Geometry check sheet. Reference: the model listing, model coordinates, mm. A direction names the side the tool comes from. Give positions to 0.01 mm unless a question says otherwise; leave off trailing zeros. Write each loop counter-clockwise with the first axis right and the second up, starting at its lowest first coordinate (ties: lowest second). Pieces come first, ordered by that corner, then holes. Notation, with made-up numbers: (81, 65.5) - (129, 65.5) arc R23 cw to (129, 88.5) - close; hole circle Ø2 at (71, 57.5). An arc over 180 degrees is marked (long way). Use a Markdown table: item, result.
```python
from build123d import *

# Parameters (mm, degrees)
CROQUIS1_R              = 4
CROQUIS1_R_2            = 2.5
CROQUIS1_R_3            = 1.5
SALIENTE_EXTRUIR1_DEPTH = 5.5
CORTAR_EXTRUIR1_DEPTH   = 10
REDONDEO1_R             = 10


with BuildPart() as part:
    # Croquis1 → Saliente-Extruir1 (new body)
    with BuildSketch(Plane.XY):
        with BuildLine():
            ThreePointArc((13.175908043, 16.287969402), (20.207859701, 17.03070481), (19.465124293, 24.062656467))
            Line((19.465124293, 24.062656467), (1.886764875, 38.28240612))
            ThreePointArc((1.886764875, 38.28240612), (1.000695169, 38.778181249), (0, 38.95))
            Line((0, 38.95), (-14, 38.95))
            ThreePointArc((-14, 38.95), (-15.75421382, 38.383666755), (-16.84611457, 36.898489248))
            Line((-16.84611457, 36.898489248), (-19.121320344, 30.071320344))
            ThreePointArc((-19.121320344, 30.071320344), (-19.771638598, 29.098050297), (-20, 27.95))
            Line((-20, 27.95), (-20, 23.95))
            ThreePointArc((-20, 23.95), (-19.121320344, 21.828679656), (-17, 20.95))
            Line((-17, 20.95), (-5, 20.95))
            ThreePointArc((-5, 20.95), (-0.298863721, 15.958939945), (4.964272191, 20.353341289))
            ThreePointArc((4.964272191, 20.353341289), (9.295071106, 18.775093958), (13.175908043, 16.287969402))
        make_face()
        with Locations((0, 20.95)):
            Circle(CROQUIS1_R, mode=Mode.SUBTRACT)
        with Locations((-15, 25.95)):
            Circle(CROQUIS1_R_2, mode=Mode.SUBTRACT)
        with Locations((0, 35.95)):
            Circle(CROQUIS1_R_3, mode=Mode.SUBTRACT)
        with Locations((-14, 35.95)):
            Circle(CROQUIS1_R_3, mode=Mode.SUBTRACT)
    extrude(amount=SALIENTE_EXTRUIR1_DEPTH)

    # Croquis2 → Cortar-Extruir1 (cut)
    with BuildSketch(Plane.XY.offset(5.5)):
        with BuildLine():
            Line((12.087138576, 30.030967124), (6.52630373, 19.907532736))
            ThreePointArc((6.52630373, 19.907532736), (10.015967096, 18.400622357), (13.175908043, 16.287969402))
            ThreePointArc((13.175908043, 16.287969402), (20.207859701, 17.03070481), (19.465124293, 24.062656467))
            Line((19.465124293, 24.062656467), (12.087138576, 30.030967124))
        make_face()
    extrude(amount=-CORTAR_EXTRUIR1_DEPTH, mode=Mode.SUBTRACT)

    # Redondeo1
    redondeo1_edges = [part.edges().sort_by_distance(p)[0] for p in [
        (12.087138576, 30.030967124, 2.75),
    ]]
    fillet(redondeo1_edges, radius=REDONDEO1_R)


solid = part.part
```
1) Mould release check, pull along Y, two halves, no side actions. Record for faces 4 (the cylindrical face through (-0.195, 37.437, 2.712)), 5 (the flat face through (-7, 38.95, 3)), 6 (the cylindrical face through (9.127, 29.349, 2.712)): pulls with the +Y half, pulls with the -Y half, needs draft (parallel to the pull), parting line crosses it, or undercut.
Working result:
| item | result |
|---|---|
| face 4 | undercut |
| face 5 | pulls with the +Y half |
| face 6 | parting line crosses it |
2) Material ranges on L1, parallel to Y at x = 0, z = 3.6; L2, parallel to Y at x = -14, z = 2.1; L3, parallel to X at y = 35.75, z = 4.75, recorded low to high. Write a range as from..to.
Working result:
| item | result |
|---|---|
| L1 | y = 15.95..16.95, 24.95..34.45, 37.45..38.95 |
| L2 | y = 20.95..23.66, 28.24..34.45, 37.45..38.95 |
| L3 | x = -17.23..-15.49, -12.51..-1.49, 1.49..5.02 |
3) Set-up check for faces 1 (the flat face through (-17.97, 33.53, 2.71)), 2 (the cylindrical face through (5.74, 20.15, 2.71)), 3 (the flat face through (-11, 20.95, 3)): record each of +Z, -Z, +X, -X, +Y, -Y from which the full face is reachable in a straight line by a thin tool's end or side.
Working result:
| item | result |
|---|---|
| face 1 | +Z, -Z, -X, +Y |
| face 2 | +Z, -Z, -Y |
| face 3 | +Z, -Z, -X, -Y |
4) Depth check by flat-ended pin: P1, Ø1.6, axis at x = -10, z = 3.5, coming from the -Y side; P2, Ø3, axis at x = -6, z = 2.5, coming from the -Y side; P3, Ø2, axis at x = -2.5, z = 3, coming from the -Y side. Enter the tip coordinate at first touch or a pass-through.
Working result:
| item | result |
|---|---|
| P1 | stops at y = 20.95 |
| P2 | stops at y = 18.77 |
| P3 | stops at y = 16.18 |
5) Section check A-A on z = 4.6. Record the boundary of the cut face in (x, y), then the cut area to 3 significant figures.
Working result:
| item | result |
|---|---|
| outline | (-20, 23.95) arc R3 ccw to (-17, 20.95) - (-5, 20.95) arc R5 ccw to (4.96, 20.35) arc R20.95 cw to (6.53, 19.91) - (8.06, 22.7) arc R10 ccw to (5.59, 35.29) - (1.89, 38.28) arc R3 ccw to (0, 38.95) - (-14, 38.95) arc R3 ccw to (-16.85, 36.9) - (-19.12, 30.07) arc R3 ccw to (-20, 27.95) - close; hole circle Ø5 at (-15, 25.95); hole circle Ø3 at (-14, 35.95); hole circle Ø8 at (0, 20.95); hole circle Ø3 at (0, 35.95) |
| area | 424 mm² |
6) Section check B-B on y = 25.95. Record the boundary of the cut face in (x, z).
Working result:
| item | result |
|---|---|
| outline | (-20, 0) - (-17.5, 0) - (-17.5, 5.5) - (-20, 5.5) - close; (-12.5, 0) - (9.17, 0) - (9.17, 5.5) - (-12.5, 5.5) - close |
7) Section check C-C on x = -11. Record the boundary of the cut face in (y, z), then the cut area to 3 significant figures.
Working result:
| item | result |
|---|---|
| outline | (20.95, 0) - (38.95, 0) - (38.95, 5.5) - (20.95, 5.5) - close |
| area | 99.0 mm² |
8) Section check D-D on y = 35.95. Record the boundary of the cut face in (x, z).
Working result:
| item | result |
|---|---|
| outline | (-17.16, 0) - (-15.5, 0) - (-15.5, 5.5) - (-17.16, 5.5) - close; (-12.5, 0) - (-1.5, 0) - (-1.5, 5.5) - (-12.5, 5.5) - close; (1.5, 0) - (4.77, 0) - (4.77, 5.5) - (1.5, 5.5) - close |
